Verification items for this drawing (mm, ordinates from the low corner). Round coordinates to 2 decimals unless told otherwise and drop trailing zeros. Order: outer loops, then holes, each group sorted by start corner. A loop starts at its lowest first (then second) coordinate and runs counter-clockwise, first axis right, second up. Notation, with made-up numbers: (71, 27.25) -> (94, 27.25) arc R29 cw to (94, 60.25) -> close; hole circle Ø6 at (17.25, 33.5). An arc over 180 degrees is marked (long way). Answer in a Markdown table with one row per item. Add a question column.
1. Material ranges on L1, parallel to X at y = 4, z = 1.25; L2, parallel to Y at x = 3, z = 1.9; L3, parallel to Y at x = 4.75, z = 0.4, recorded low to high. Write a range as from..to.
2. Sectioned sample at C-C, the plane x = 2.5. Record the boundary of the cut face in (y, z).
3. Depth check by flat-ended pin: P1, Ø1.5, axis at x = 3, z = 2.5, coming from the +Y side (1 decimal); P2, Ø1.5, axis at x = 3.5, z = 3, coming from the -Y side. Enter the tip coordinate at first touch or a pass-through.
4. Draft check along X on the marked faces 1, 2, 3 and 4. Enter one of: +X half, -X half, draft (parallel to the pull), parting line (faces both ways), or undercut.
5. Sectioned sample at B-B, the plane z = 3.9. Record the boundary of the cut face in (x, y), then the cut area to 3 significant figures.
6. Sectioned sample at A-A, the plane y = 5. Record the boundary of the cut face in (x, z).
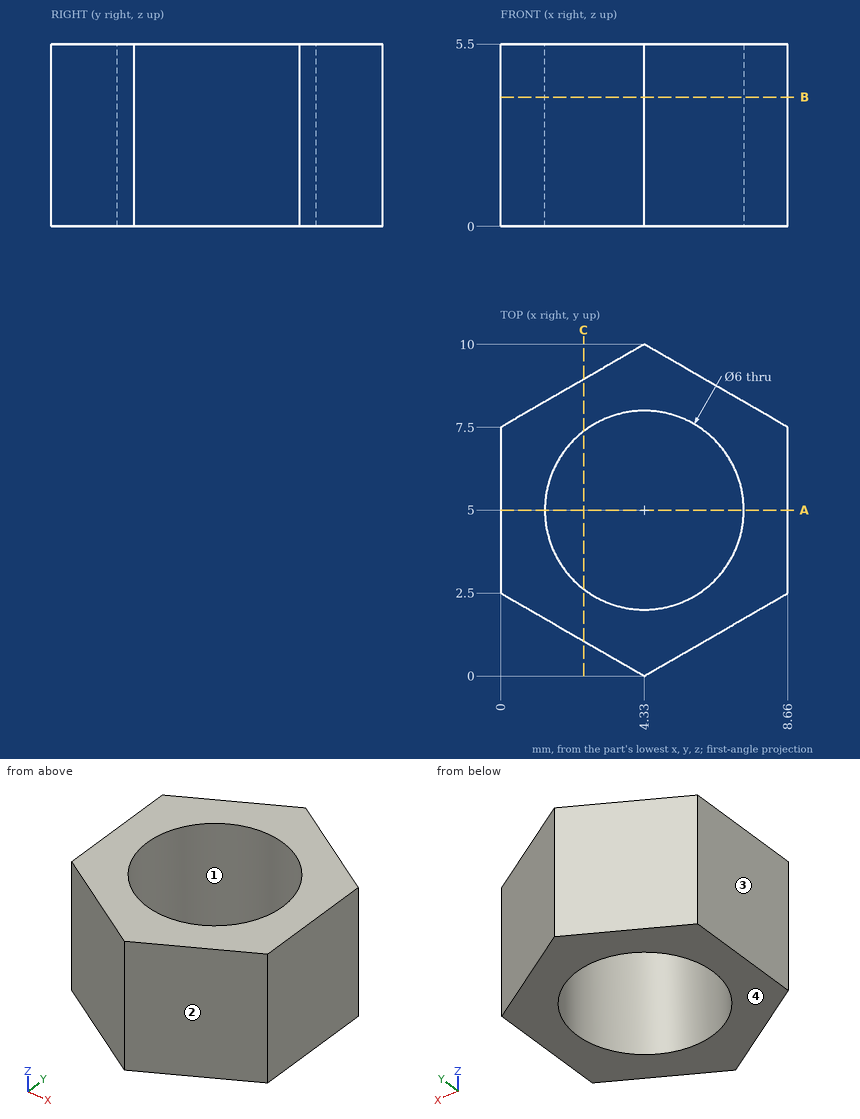
Answer key:
| question | item | result |
|---|---|---|
| 1 | L1 | x = 0..1.5, 7.16..8.66 |
| 1 | L2 | y = 0.77..2.31, 7.69..9.23 |
| 1 | L3 | y = 0.24..2.03, 7.97..9.76 |
| 2 | outline | (1.06, 0) -> (2.62, 0) -> (2.62, 5.5) -> (1.06, 5.5) -> close; (7.38, 0) -> (8.94, 0) -> (8.94, 5.5) -> (7.38, 5.5) -> close |
| 3 | P1 | stops at y = 9.7 |
| 3 | P2 | stops at y = 0.05 |
| 4 | face 1 | undercut |
| 4 | face 2 | +X half |
| 4 | face 3 | -X half |
| 4 | face 4 | draft |
| 5 | outline | (0, 2.5) -> (4.33, 0) -> (8.66, 2.5) -> (8.66, 7.5) -> (4.33, 10) -> (0, 7.5) -> close; hole circle Ø6 at (4.33, 5) |
| 5 | area | 36.7 mm² |
| 6 | outline | (0, 0) -> (1.33, 0) -> (1.33, 5.5) -> (0, 5.5) -> close; (7.33, 0) -> (8.66, 0) -> (8.66, 5.5) -> (7.33, 5.5) -> close |
